Job drawing, mm, ordinate dimensions from the low corner. One solid piece. A direction names the side the tool comes from. Round coordinates to 2 decimals unless told otherwise and drop trailing zeros. Write each loop counter-clockwise with the first axis right and the second up, starting at its lowest first coordinate (ties: lowest second). Pieces come first, ordered by that corner, then holes.
1) Saw through at C-C (y = 11.75). Write the cut outline in (x, z), plus the area to 3 significant figures.
2) Which spindle directions (+Z, -Z, +X, -X, +Y, -Y) get a long thin tool onto all of the face, cutting with end or side? Do the marked faces 1 and 2. Say none if no direction does.
3) Pull direction X, two halves, no side cores. Call the marked faces 3, 4 and 5: +X half, -X half, draft (parallel to the pull), parting line (faces both ways), or undercut.
4) Flat gauge pin, fed straight in: pin 1 (4 mm diameter, centred on x = 30, y = 7.5, fed in from +Z). Where does the tip first touch, or does it go through?
5) Wall check: probe 1 along X at (y, z) = (14, 2.25); probe 2 along X at (y, z) = (8.5, 6.75); probe 3 along Y at (x, z) = (33.5, 0.5). Give the ranges that are in metal, low to high.
6) Saw through at B-B (z = 7.25). Write the cut outline in (x, y).
7) Saw through at A-A (y = 20.75). Write the cut outline in (x, z), plus the area to 3 significant figures.
8) Saw through at D-D (x = 27). Write the cut outline in (y, z).
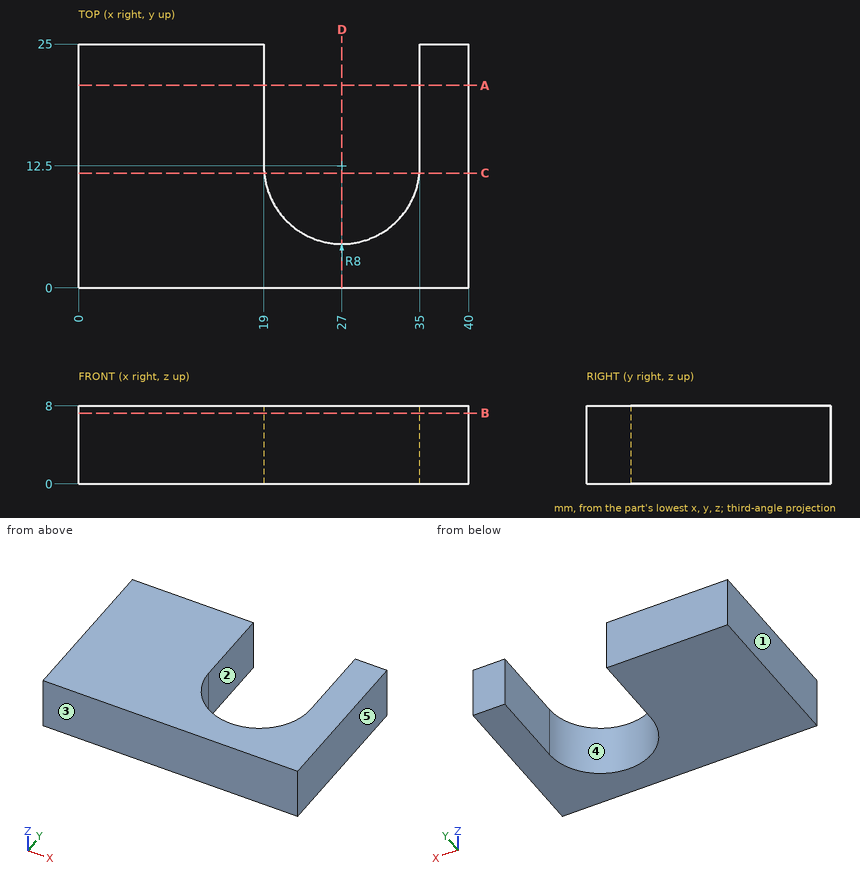
Evaluation:
1. outline: (0, 0) - (19.04, 0) - (19.04, 8) - (0, 8) - close; (34.96, 0) - (40, 0) - (40, 8) - (34.96, 8) - close
1. area: 193 mm2
2. face 1: +Z, -Z, -X, +Y, -Y
2. face 2: +Z, -Z, +Y
3. face 3: draft
3. face 4: undercut
3. face 5: +X half
4. pin 1: passes through
5. probe 1: x = 0 to 19, 35 to 40
5. probe 2: x = 0 to 20.07, 33.93 to 40
5. probe 3: y = 0 to 7.84
6. outline: (0, 0) - (40, 0) - (40, 25) - (35, 25) - (35, 12.5) arc R8 cw to (19, 12.5) - (19, 25) - (0, 25) - close
7. outline: (0, 0) - (19, 0) - (19, 8) - (0, 8) - close; (35, 0) - (40, 0) - (40, 8) - (35, 8) - close
7. area: 192 mm2
8. outline: (0, 0) - (4.5, 0) - (4.5, 8) - (0, 8) - close
